```python
from build123d import *

# Parameters (mm, degrees)
F1_DEPTH = 5.08
F2_R     = 4.445
F3_DEPTH = 2.032
F5_D     = 5


with BuildPart() as f1:
    # F0 (on Top) → F1 (new body)
    with BuildSketch(Plane.XY):
        Polygon((3.3457980823, 5.6883025765), (-3.2533154946, 5.7416974235), (-6.5991135768, 0.0533948469), (-3.3457980823, -5.6883025765), (3.2533154946, -5.7416974235), (6.5991135768, -0.0533948469), align=None)
    extrude(amount=F1_DEPTH)

    # F2 (on face) → F3 (join)
    with BuildSketch(Plane(origin=(0, 0, 0), x_dir=(1, 0, 0), z_dir=(0, 0, -1))):
        Circle(F2_R)
    extrude(amount=F3_DEPTH)

    # F5 (through all)
    with Locations(Plane(origin=(0, 0, -2.032), x_dir=(1, 0, 0), z_dir=(0, 0, -1))):
        with Locations((0, 0)):
            Hole(F5_D / 2)


solid = f1.part
```
The model under review builds one solid part; all positions refer to its coordinate system, in mm. A direction names the side the tool comes from. Coordinates: 2 decimals unless noted, no trailing zeros. Write each loop counter-clockwise with the first axis right and the second up, starting at its lowest first coordinate (ties: lowest second). Pieces come first, ordered by that corner, then holes. Notation, with made-up numbers: (84.5, 85.25) -> (91.5, 85.25) arc R19 cw to (91.5, 103.25) -> close; hole circle Ø11 at (-15.75, -14.5). An arc over 180 degrees is marked (long way). One line per item, written item: value. Start each with the question number.
Q1. Add section A-A, the plane z = 2.25. Give the boundary of the cut face in (x, y), then the cut area to 3 significant figures.
Q2. Add section B-B, the plane x = 0. Give the boundary of the cut face in (y, z) (3 decimals).
Q3. The part is to be moulded in two halves that separate along Y. For faces 3 (the face through (-0.96, 4.34, -1)), 4 (the face through (3, 0, 5.08)), 5 (the face through (4.9, -2.94, 2.5)), 6 (the face through (0.54, 2.44, 1.57)), say which applies: +Y half, -Y half, draft (parallel to the pull), parting line (faces both ways), or undercut.
Q4. For faces 1 (the face through (-4.995, -2.777, 2.504)), 2 (the face through (1.9, 4.3, 0)), list the 3-axis set-ups (+Z, -Z, +X, -X, +Y, -Y) from which the entire face can be reached by the end or side of a thin tool; tool diameter is ignored.
Q5. To check wall thickness, follow probe 1 along Y at (x, z) = (0, 0.5); probe 2 along Z at (x, y) = (2.5, 4.75); probe 3 along Y at (x, z) = (1, 3). State the ranges of each line that lie inside material, in increasing order.
Q6. Add section C-C, the plane y = -1.75. Give the boundary of the cut face in (x, z).
Q7. Clearance check with flat-ended pins moving along their axes: P1, Ø4, axis at y = -3.5, z = -1, coming from the +X side; P2, Ø1.5, axis at x = -4, z = -1, coming from the -Y side. State where each tip first meets the part, or that it passes through.
Q8. Add section D-D, the plane y = -3.75. Give the boundary of the cut face in (x, z), then the cut area to 3 significant figures.
Response:
1. outline: (-6.6, 0.05) -> (-3.35, -5.69) -> (3.25, -5.74) -> (6.6, -0.05) -> (3.35, 5.69) -> (-3.25, 5.74) -> close; hole circle Ø5 at (0, 0)
1. area: 93.5 mm²
2. outline: (-5.715, 0) -> (-4.445, 0) -> (-4.445, -2.032) -> (-2.5, -2.032) -> (-2.5, 5.08) -> (-5.715, 5.08) -> close; (2.5, -2.032) -> (4.445, -2.032) -> (4.445, 0) -> (5.715, 0) -> (5.715, 5.08) -> (2.5, 5.08) -> close
3. face 3: parting line
3. face 4: draft
3. face 5: -Y half
3. face 6: undercut
4. face 1: +Z, -Z, -X, -Y
4. face 2: -Z
5. probe 1: -5.72 to -2.5, 2.5 to 5.72
5. probe 2: 0 to 5.08
5. probe 3: -5.72 to -2.29, 2.29 to 5.71
6. outline: (-5.58, 0) -> (-4.09, 0) -> (-4.09, -2.03) -> (-1.79, -2.03) -> (-1.79, 5.08) -> (-5.58, 5.08) -> close; (1.79, -2.03) -> (4.09, -2.03) -> (4.09, 0) -> (5.6, 0) -> (5.6, 5.08) -> (1.79, 5.08) -> close
7. P1: x = 5.59
7. P2: y = -3.03
8. outline: (-4.44, 0) -> (-2.39, 0) -> (-2.39, -2.03) -> (2.39, -2.03) -> (2.39, 0) -> (4.42, 0) -> (4.42, 5.08) -> (-4.44, 5.08) -> close
8. area: 54.8 mm²
